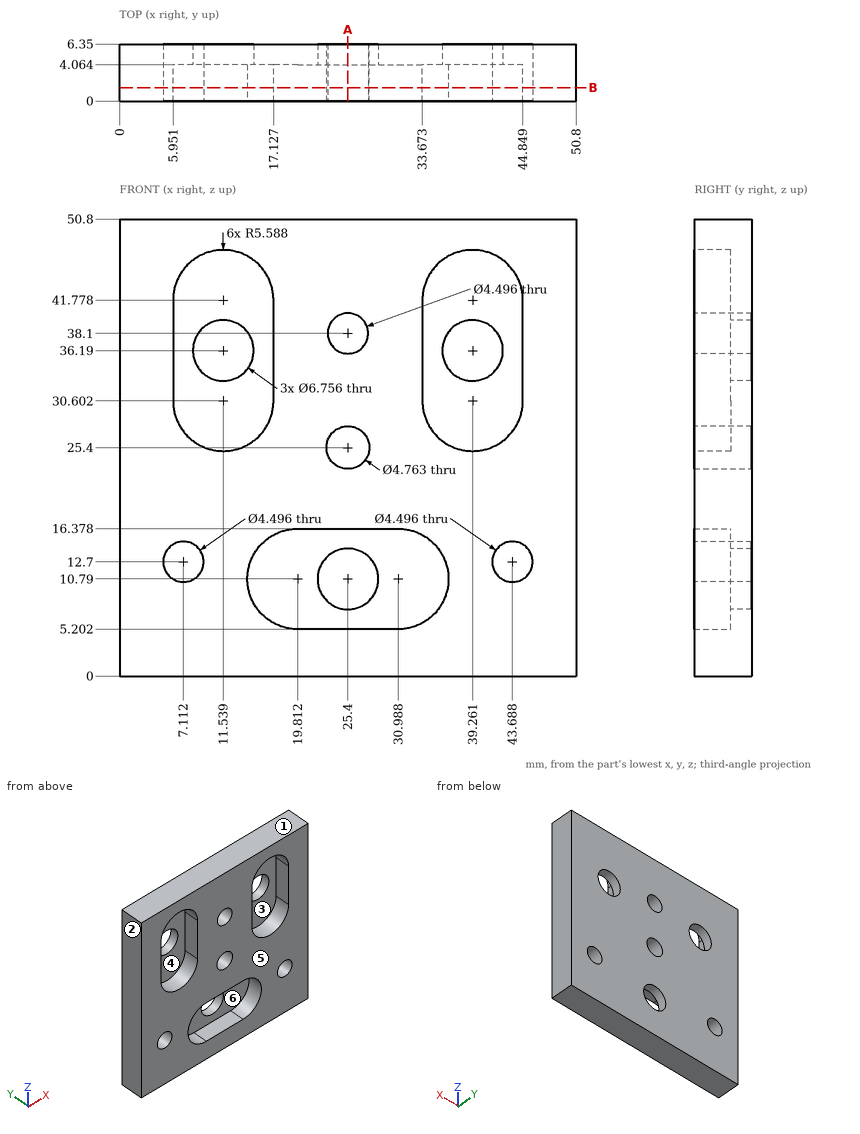
Print and shaded views of the part. All mm, measured from the part's lowest x, y and z. A direction names the side the tool comes from. Round coordinates to 2 decimals unless told otherwise and drop trailing zeros. Write each loop counter-clockwise with the first axis right and the second up, starting at its lowest first coordinate (ties: lowest second). Pieces come first, ordered by that corner, then holes. Notation, with made-up numbers: (74.25, 75.25) - (103.25, 75.25) arc R28 ccw to (103.25, 95.25) - close; hole circle Ø1 at (17.5, 26). An arc over 180 degrees is marked (long way). Write each question's results on one line, items separated by ' | '. Start each with the question number.
Item 1: Saw through at A-A (x = 25.4). State how many separate pieces and enclosed holes the cut face has, and give its area (3 significant figures).
Item 2: Drop a flat-ended pin along its axis: P1, Ø5.5, axis at x = 39.5, z = 35, coming from the -Y side. Give the stop position or say it passes through.
Item 3: Wall check: L1, parallel to X at y = 1, z = 12 (1 decimal); L2, parallel to Z at x = 27, y = 3.5 (1 decimal); L3, parallel to Z at x = 23.5, y = 1.75 (1 decimal). Give the ranges that are in metal, low to high. Write a range as [from, to].
Item 4: Mould opens along Z. For the marked faces 1, 2, 3 and 4 say: pulls with the +Z half, pulls with the -Z half, needs draft (parallel to the pull), parting line crosses it, or undercut.
Item 5: Which spindle directions (+Z, -Z, +X, -X, +Y, -Y) get a long thin tool onto all of the face, cutting with end or side? Do the marked faces 5 and 6. Say none if no direction does.
Item 6: Saw through at B-B (y = 1.5). Write the cut outline in (x, z) (1 decimal), and give its area (3 significant figures).
Results are:
1) separate pieces: 4 | enclosed holes: 0 | area: 203 mm²
2) P1: stops at y = 4.06
3) L1: x = [0, 5], [9.2, 14.4], [36.4, 41.6], [45.8, 50.8] | L2: z = [0, 5.2], [16.4, 23.6], [27.2, 36.5], [39.7, 50.8] | L3: z = [0, 5.2], [16.4, 24], [26.8, 36.9], [39.3, 50.8]
4) face 1: pulls with the +Z half | face 2: needs draft | face 3: undercut | face 4: undercut
5) face 5: +Z, -Z, +X, -X, -Y | face 6: -Y
6) outline: (0, 0) - (50.8, 0) - (50.8, 50.8) - (0, 50.8) - close; hole circle Ø4.5 at (7.1, 12.7); hole (6, 30.6) arc R5.6 ccw to (17.1, 30.6) - (17.1, 41.8) arc R5.6 ccw to (6, 41.8) - close; hole (19.8, 5.2) - (31, 5.2) arc R5.6 ccw to (31, 16.4) - (19.8, 16.4) arc R5.6 ccw to start; hole circle Ø4.8 at (25.4, 25.4); hole circle Ø4.5 at (25.4, 38.1); hole (33.7, 30.6) arc R5.6 ccw to (44.8, 30.6) - (44.8, 41.8) arc R5.6 ccw to (33.7, 41.8) - close; hole circle Ø4.5 at (43.7, 12.7) | area: 1,850 mm²
